```python
from build123d import *

# Parameters (mm, degrees)
SALIENTE_EXTRUIR1_DEPTH = 15
CROQUIS2_R              = 6
CORTAR_EXTRUIR1_DEPTH   = 104.918297485


with BuildPart() as part:
    # Croquis1 → Saliente-Extruir1 (new body)
    with BuildSketch(Plane.XY):
        with BuildLine():
            Line((-64.346717088, 45.961940777), (-52.620489657, 34.235713346))
            ThreePointArc((-52.620489657, 34.235713346), (-51.206737587, 31.410509176), (-51.768834222, 28.301727921))
            ThreePointArc((-51.768834222, 28.301727921), (-58.508070764, -7.603003058), (-42.816126208, -40.592848343))
            ThreePointArc((-42.816126208, -40.592848343), (-41.896840908, -50.430118648), (-51.234753159, -53.658178023))
            ThreePointArc((-51.234753159, -53.658178023), (-66.988640567, -63.012773757), (-55.154328933, -77))
            Line((-55.154328933, -77), (55.154328933, -77))
            ThreePointArc((55.154328933, -77), (66.988640567, -63.012773757), (51.234753159, -53.658178023))
            ThreePointArc((51.234753159, -53.658178023), (41.896840908, -50.430118648), (42.816126208, -40.592848343))
            ThreePointArc((42.816126208, -40.592848343), (58.508070764, -7.603003058), (51.768834222, 28.301727921))
            ThreePointArc((51.768834222, 28.301727921), (51.206737587, 31.410509176), (52.620489657, 34.235713346))
            Line((52.620489657, 34.235713346), (64.346717088, 45.961940777))
            ThreePointArc((64.346717088, 45.961940777), (64.346717088, 64.346717088), (45.961940777, 64.346717088))
            Line((45.961940777, 64.346717088), (34.235713346, 52.620489657))
            ThreePointArc((34.235713346, 52.620489657), (31.410509176, 51.206737587), (28.301727921, 51.768834222))
            ThreePointArc((28.301727921, 51.768834222), (0, 59), (-28.301727921, 51.768834222))
            ThreePointArc((-28.301727921, 51.768834222), (-31.410509176, 51.206737587), (-34.235713346, 52.620489657))
            Line((-34.235713346, 52.620489657), (-45.961940777, 64.346717088))
            ThreePointArc((-45.961940777, 64.346717088), (-64.346717088, 64.346717088), (-64.346717088, 45.961940777))
        make_face()
    extrude(amount=SALIENTE_EXTRUIR1_DEPTH)

    # Croquis2 → Cortar-Extruir1 (cut, through all)
    with BuildSketch(Plane.XY.offset(15)):
        with Locations((-55.154328933, 55.154328933)):
            Circle(CROQUIS2_R)
        with Locations((55.154328933, 55.154328933)):
            Circle(CROQUIS2_R)
        with Locations((-55.154328933, -65)):
            Circle(CROQUIS2_R)
        with Locations((55.154328933, -65)):
            Circle(CROQUIS2_R)
        with BuildLine():
            Line((-8, 43), (-8, 25.787593916))
            ThreePointArc((-8, 25.787593916), (-10.332452674, 24.944747378), (-12.577728279, 23.891436778))
            Line((-12.577728279, 23.891436778), (-24.748737342, 36.062445841))
            ThreePointArc((-24.748737342, 36.062445841), (-36.062445841, 36.062445841), (-36.062445841, 24.748737342))
            Line((-36.062445841, 24.748737342), (-23.891436778, 12.577728279))
            ThreePointArc((-23.891436778, 12.577728279), (-24.944747378, 10.332452674), (-25.787593916, 8))
            Line((-25.787593916, 8), (-43, 8))
            ThreePointArc((-43, 8), (-51, 0), (-43, -8))
            Line((-43, -8), (-25.787593916, -8))
            ThreePointArc((-25.787593916, -8), (-24.944747378, -10.332452674), (-23.891436778, -12.577728279))
            Line((-23.891436778, -12.577728279), (-36.062445841, -24.748737342))
            ThreePointArc((-36.062445841, -24.748737342), (-36.062445841, -36.062445841), (-24.748737342, -36.062445841))
            Line((-24.748737342, -36.062445841), (-12.577728279, -23.891436778))
            ThreePointArc((-12.577728279, -23.891436778), (-10.332452674, -24.944747378), (-8, -25.787593916))
            Line((-8, -25.787593916), (-8, -43))
            ThreePointArc((-8, -43), (0, -51), (8, -43))
            Line((8, -43), (8, -25.787593916))
            ThreePointArc((8, -25.787593916), (10.332452674, -24.944747378), (12.577728279, -23.891436778))
            Line((12.577728279, -23.891436778), (24.748737342, -36.062445841))
            ThreePointArc((24.748737342, -36.062445841), (36.062445841, -36.062445841), (36.062445841, -24.748737342))
            Line((36.062445841, -24.748737342), (23.891436778, -12.577728279))
            ThreePointArc((23.891436778, -12.577728279), (24.944747378, -10.332452674), (25.787593916, -8))
            Line((25.787593916, -8), (43, -8))
            ThreePointArc((43, -8), (51, 0), (43, 8))
            Line((43, 8), (25.787593916, 8))
            ThreePointArc((25.787593916, 8), (24.944747378, 10.332452674), (23.891436778, 12.577728279))
            Line((23.891436778, 12.577728279), (36.062445841, 24.748737342))
            ThreePointArc((36.062445841, 24.748737342), (36.062445841, 36.062445841), (24.748737342, 36.062445841))
            Line((24.748737342, 36.062445841), (12.577728279, 23.891436778))
            ThreePointArc((12.577728279, 23.891436778), (10.332452674, 24.944747378), (8, 25.787593916))
            Line((8, 25.787593916), (8, 43))
            ThreePointArc((8, 43), (0, 51), (-8, 43))
        make_face()
    extrude(amount=-CORTAR_EXTRUIR1_DEPTH, mode=Mode.SUBTRACT)


solid = part.part
```
Work out the finished part from the listing and answer in its coordinate system (mm). A direction names the side the tool comes from. Give positions to 0.01 mm unless a question says otherwise; leave off trailing zeros. Write each loop counter-clockwise with the first axis right and the second up, starting at its lowest first coordinate (ties: lowest second). Pieces come first, ordered by that corner, then holes.
(1) The part is cut by section B-B on x = 0. Write down the section's boundary in (y, z).
Final values:
outline: (-77, 0) - (-51, 0) - (-51, 15) - (-77, 15) - close; (51, 0) - (59, 0) - (59, 15) - (51, 15) - close
(2) Straight lines are drawn through the part: line 1 (X direction, y = 32.5, z = 4.75); line 2 (Y direction, x = -30, z = 9.25); line 3 (X direction, y = -66, z = 6.75). For each, find the intervals that lie inside material, in ascending order.
Final values:
line 1: x = -51.49 to -38.13, -21.19 to -8, 8 to 21.19, 38.13 to 51.49
line 2: y = -77 to -38.4, -18.69 to -8, 8 to 18.69, 38.4 to 51.21
line 3: x = -67.11 to -61.07, -49.24 to 49.24, 61.07 to 67.11
(3) Which of the six approach directions +Z, -Z, +X, -X, +Y, -Y give full straight-line access (tool end or side, diameter ignored) to faces 4 (the cylindrical face through (-24.96, -10.3, 7.6)), 5 (the flat face through (-1, -77, 7)), 6 (the flat face through (-40.017, 58.402, 7.395))?
Final values:
face 4: +Z, -Z
face 5: +Z, -Z, +X, -X, -Y
face 6: +Z, -Z, +Y
(4) The part is cut by section A-A on y = -65. Write down the section's boundary in (x, z), plus the area to 3 significant figures.
Final values:
outline: (-67.15, 0) - (-61.15, 0) - (-61.15, 15) - (-67.15, 15) - close; (-49.15, 0) - (49.15, 0) - (49.15, 15) - (-49.15, 15) - close; (61.15, 0) - (67.15, 0) - (67.15, 15) - (61.15, 15) - close
area: 1,650 mm2
(5) The mould has two halves that part along X. Classify faces 1 (the cylindrical face through (51.2, 31.37, 7.4)), 2 (the flat face through (-31.2, -19.5, 15)), 3 (the cylindrical face through (-49.431, 56.957, 7.605)): pulls with the +X half, pulls with the -X half, needs draft (parallel to the pull), parting line crosses it, or undercut.
Final values:
face 1: pulls with the +X half
face 2: needs draft
face 3: undercut
(6) Flat-ended cylindrical pins translate along their axes: pin 1 Ø4.5 at (x, z) = (-30.5, 5) entering from +Y; pin 2 Ø2 at (y, z) = (-40, 3.5) entering from +X; pin 3 Ø4 at (x, z) = (-38, 3) entering from +Y; pin 4 Ø19 at (x, y) = (-55.15, 55.15) entering from -Z. Find the tip coordinate at first contact, or state that the pin passes through.
Final values:
pin 1: stops at y = 51.8
pin 2: stops at x = 44.27
pin 3: stops at y = 58.38
pin 4: stops at z = 0
(7) The part is cut by section C-C on y = 0. Write down the section's boundary in (x, z), plus the area to 3 significant figures.
Final values:
outline: (-59, 0) - (-51, 0) - (-51, 15) - (-59, 15) - close; (51, 0) - (59, 0) - (59, 15) - (51, 15) - close
area: 240 mm2
(8) The part is cut by section D-D on y = 31.5. Write down the section's boundary in (x, z), plus the area to 3 significant figures.
Final values:
outline: (-51.22, 0) - (-38.33, 0) - (-38.33, 15) - (-51.22, 15) - close; (-20.19, 0) - (-8, 0) - (-8, 15) - (-20.19, 15) - close; (8, 0) - (20.19, 0) - (20.19, 15) - (8, 15) - close; (38.33, 0) - (51.22, 0) - (51.22, 15) - (38.33, 15) - close
area: 752 mm2
